Part model, mm, in its own coordinate system. A direction names the side the tool comes from. Round coordinates to 2 decimals unless told otherwise and drop trailing zeros. Order: outer loops, then holes, each group sorted by start corner. A loop starts at its lowest first (then second) coordinate and runs counter-clockwise, first axis right, second up. Notation, with made-up numbers: (52.5, 19) - (98.5, 19) arc R21 cw to (98.5, 33) - close; hole circle Ø4 at (83.5, 76.5). An arc over 180 degrees is marked (long way). Return JSON: item names as keys, results as strings. Group by question number.
Item 1: Saw through at B-B on z = 9. List the corners of the cut face in (x, y), and give its area (3 significant figures).
Item 2: Saw through at C-C on y = 139.5. List the corners of the cut face in (x, z), and give its area (3 significant figures).
Item 3: Drop flat-ended pins along their axis: pin 1 (2 mm diameter, centred on x = -191.5, y = 134, fed in from +Z); pin 2 (2 mm diameter, centred on x = -191, z = 6.5, fed in from -Y); pin 3 (1 mm diameter, centred on x = -191.5, y = 138.5, fed in from +Z); pin 4 (3 mm diameter, centred on x = -187, z = 4.5, fed in from -Y). Give the stop position or say it passes through.
Item 4: Saw through at D-D on x = -188.5. List the corners of the cut face in (y, z), and give its area (3 significant figures).
Item 5: Saw through at A-A on x = -187. List the corners of the cut face in (y, z), and give its area (3 significant figures).
Item 6: Tool access for faces 1 (the face through (-187.037, 140.076, 3.536)), 2 (the face through (-185.72, 141.89, 11.16)), 3 (the face through (-192.2, 133, 0.5)): list every direction of +Z, -Z, +X, -X, +Y, -Y with a clear straight run to the whole face (end or side of a thin tool).
Item 7: Two-plate mould, pull along Z, no slides. Class faces 4 (the face through (-190.4, 135.44, 2.77)), 5 (the face through (-192.3, 132.9, 11.5)), 6 (the face through (-187.02, 140.1, 8.33)): released by +Z, released by -Z, zero draft, split by the parting line, or undercut.
Item 8: Probe probe 1 along Z at (x, y) = (-188, 139); probe 2 along Y at (x, z) = (-186.5, 1.25); probe 3 along Y at (x, z) = (-192, 11.25). List the from-to ranges inside material, lowest first.
```python
from build123d import *

# Parameters (mm, degrees)
BOX232_W                  = 0.5
BOX232_H                  = 1
BOX232_DEPTH              = 15
BOX232_ROLL_ANGLE         = 46
BOX233_W                  = 0.5
BOX233_H                  = 1
BOX233_DEPTH              = 15
BOX233_ROLL_ANGLE         = -46
BOX231_W                  = 0.5
BOX231_H                  = 1
BOX231_DEPTH              = 11
FUSION020_PLACEMENT_ANGLE = -36


with BuildPart() as cubo232:
    # Box232 → Box232 (new body)
    with BuildSketch(Plane.XY):
        with Locations((0.25, 0.5)):
            Rectangle(BOX232_W, BOX232_H)
    extrude(amount=BOX232_DEPTH)


with BuildPart() as cubo232_1:
    # Box232 roll: moved
    add(cubo232.part.rotate(Axis((0, 0, 0), (1, 0, 0)), BOX232_ROLL_ANGLE))


with BuildPart() as cubo232_2:
    # Box232 placement: moved
    add(cubo232_1.part.moved(Location((0, 11, 0.5))))


with BuildPart() as cubo233:
    # Box233 → Box233 (new body)
    with BuildSketch(Plane.XY):
        with Locations((0.25, 0.5)):
            Rectangle(BOX233_W, BOX233_H)
    extrude(amount=BOX233_DEPTH)


with BuildPart() as cubo233_1:
    # Box233 roll: moved
    add(cubo233.part.rotate(Axis((0, 0, 0), (1, 0, 0)), BOX233_ROLL_ANGLE))


with BuildPart() as cubo233_2:
    # Box233 placement: moved
    add(cubo233_1.part.moved(Location((0, 0.4, 1.1))))


with BuildPart() as fusion020:
    # Box231 → Box231 (new body)
    with BuildSketch(Plane.XY.offset(0.5)):
        with Locations((0.25, 0.5)):
            Rectangle(BOX231_W, BOX231_H)
    extrude(amount=BOX231_DEPTH)

    # Fusion020: union Cubo232, Cubo233
    add(cubo232_2.part)
    add(cubo233_2.part)


with BuildPart() as fusion020_1:
    # Fusion020 placement: moved
    add(fusion020.part.moved(Location((-192.7, 132.7, 0))).rotate(Axis((-192.7, 132.7, 0), (0, 0, 1)), FUSION020_PLACEMENT_ANGLE))


solid = fusion020_1.part
```
Filled in:
{
 "1": {"outline": "(-192.7, 132.7) - (-192.3, 132.41) - (-191.71, 133.22) - (-192.11, 133.51) - close; (-191.41, 134.48) - (-191, 134.18) - (-190.16, 135.35) - (-190.56, 135.64) - close; (-187.66, 139.64) - (-187.25, 139.35) - (-186.41, 140.51) - (-186.81, 140.81) - close", "area": "1.94 mm^2"},
 "2": {"outline": "(-187.76, 3.01) - (-187.14, 2.65) - (-187.14, 4.05) - (-187.76, 4.4) - close; (-187.76, 7.44) - (-187.14, 7.79) - (-187.14, 9.18) - (-187.76, 8.83) - close", "area": "1.72 mm^2"},
 "3": {"pin 1": "stops at z = 11.64", "pin 2": "stops at y = 132.81", "pin 3": "passes through", "pin 4": "stops at y = 137.68"},
 "4": {"outline": "(137.63, 4.89) - (138.48, 4.22) - (138.48, 5.61) - (138.09, 5.92) - (138.48, 6.22) - (138.48, 7.61) - (137.63, 6.95) - close", "area": "2.20 mm^2"},
 "5": {"outline": "(139.69, 2.42) - (140.55, 1.76) - (140.55, 3.15) - (139.69, 3.81) - close; (139.69, 8.02) - (140.55, 8.69) - (140.55, 10.08) - (139.69, 9.41) - close", "area": "2.37 mm^2"},
 "6": {"face 1": "+X, +Y", "face 2": "+Z, +X, +Y", "face 3": "-Z, -X, -Y"},
 "7": {"face 4": "released by -Z", "face 5": "released by +Z", "face 6": "undercut"},
 "8": {"probe 1": "z = 3.53 to 4.92, 6.91 to 8.3", "probe 2": "y = 140.83 to 141.23", "probe 3": "y = 132.81 to 133.66"}
}
